The listing builds one solid part. Answer for the finished solid, in the listing's coordinates (mm). Face numbers are marked on the shaded views. A direction names the side the tool comes from. Round coordinates to 2 decimals unless told otherwise and drop trailing zeros. Loops run counter-clockwise (first coordinate to the right, second up) from the corner with the lowest first, then second, coordinate; pieces in that order, holes last. Notation, with made-up numbers: (51, 73) -> (86, 73) arc R16 cw to (86, 98) -> close; hole circle Ø5 at (-34.5, 19). An arc over 180 degrees is marked (long way). Use a Markdown table: item, result. Add a question column.
Q1. Which of the six approach directions +Z, -Z, +X, -X, +Y, -Y give full straight-line access (tool end or side, diameter ignored) to the marked faces 4, 5, 6 and 7?
Q2. Section C-C on x = 8 is taken. Give the vertices of the cut face in (y, z).
Q3. Section A-A on x = 0 is taken. Give the vertices of the cut face in (y, z).
Q4. For a pull along X with two mould halves and no side action, classify the marked faces 1, 2 and 3 as released by +X, released by -X, zero draft, split by the parting line, or undercut.
Q5. Section D-D on x = 3.75 is taken. Give the vertices of the cut face in (y, z).
Q6. Consider line 1 (X direction, y = 2.55, z = 14); line 2 (X direction, y = 0.85, z = 9.75); line 3 (Z direction, x = 0, y = 2.45). Determine where each line is inside the solid, lowest interval first.
Q7. Section B-B on y = 2.3 is taken. Give the vertices of the cut face in (x, z), then the cut area to 3 significant figures.
Q8. Given pin 1 Ø1.2 at (x, y) = (11.5, 1.5) entering from +Z; pin 2 Ø0.9 at (y, z) = (1, 13.5) entering from +X; pin 3 Ø0.6 at (x, y) = (0.5, 1) entering from +Z, each flat-ended and moving along its own axis, determine where each tip first touches the part or whether it passes through.
from build123d import *

# Parameters (mm, degrees)
BOSS_EXTRUDE1_DEPTH = 3
SKETCH3_R           = 1.5
CUT_EXTRUDE1_DEPTH  = 3
FILLET1_R           = 2
SKETCH4_R           = 1
CUT_EXTRUDE2_DEPTH  = 10


with BuildPart() as part:
    # Sketch2 → Boss-Extrude1 (new body)
    with BuildSketch(Plane(origin=(0, 0, 0), x_dir=(1, 0, 0), z_dir=(0, 1, 0))):
        with BuildLine():
            Line((4.668611776, -14.59443044), (4.668611776, -22.09443044))
            ThreePointArc((4.668611776, -22.09443044), (7.568611776, -24.99443044), (10.468611776, -22.09443044))
            Line((10.468611776, -22.09443044), (10.468611776, -14.59443044))
            Line((10.468611776, -14.59443044), (10.468611776, -10.59443044))
            Line((10.468611776, -10.59443044), (11.968611776, -10.59443044))
            Line((11.968611776, -10.59443044), (11.968611776, -5.761851858))
            ThreePointArc((11.968611776, -5.761851858), (7.254363967, -4.368466387), (5, 0))
            ThreePointArc((5, 0), (0, 5), (-5, 0))
            ThreePointArc((-5, 0), (-7.028472422, -4.339612176), (-11.531388224, -5.973834769))
            Line((-11.531388224, -5.973834769), (-11.531388224, -10.806413351))
            Line((-11.531388224, -10.806413351), (-10.031388224, -10.806413351))
            Line((-10.031388224, -10.806413351), (-10.031388224, -14.806413351))
            Line((-10.031388224, -14.806413351), (-4.231388224, -14.806413351))
            Line((-4.231388224, -14.806413351), (-4.231388224, -10.806413351))
            Line((-4.231388224, -10.806413351), (-0.781388224, -10.806413351))
            Line((-0.781388224, -10.806413351), (-0.781388224, -6.306413351))
            Line((-0.781388224, -6.306413351), (1.218611776, -6.306413351))
            Line((1.218611776, -6.306413351), (1.218611776, -10.806413351))
            Line((1.218611776, -10.806413351), (4.668611776, -10.806413351))
            Line((4.668611776, -10.806413351), (4.668611776, -14.59443044))
        make_face()
    extrude(amount=BOSS_EXTRUDE1_DEPTH)

    # Sketch3 → Cut-Extrude1 (cut)
    with BuildSketch(Plane(origin=(0, 3, 0), x_dir=(1, 0, 0), z_dir=(0, 1, 0))):
        Circle(SKETCH3_R)
    extrude(amount=-CUT_EXTRUDE1_DEPTH, mode=Mode.SUBTRACT)

    # Fillet1
    fillet1_edges = [part.edges().sort_by_distance(p)[0] for p in [
        (-11.531388224, 1.5, 5.973834769),
        (11.968611776, 1.5, 5.761851858),
    ]]
    fillet(fillet1_edges, radius=FILLET1_R)

    # Sketch4 → Cut-Extrude2 (cut)
    with BuildSketch(Plane(origin=(0, 3, 0), x_dir=(1, 0, 0), z_dir=(0, 1, 0))):
        with Locations((7.568611776, -22.09443044)):
            Circle(SKETCH4_R)
    extrude(amount=-CUT_EXTRUDE2_DEPTH, mode=Mode.SUBTRACT)


solid = part.part
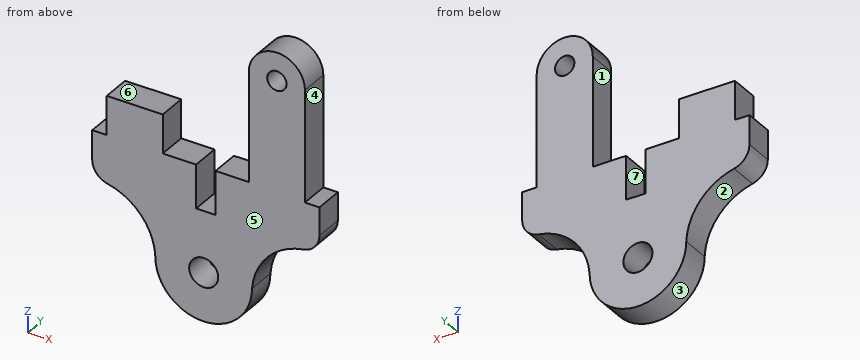
Checked values:
| question | item | result |
|---|---|---|
| 1 | face 4 | +Z, +X, +Y, -Y |
| 1 | face 5 | +Z, -Z, +X, -X, -Y |
| 1 | face 6 | +Z, -X, +Y, -Y |
| 1 | face 7 | +Z, +Y, -Y |
| 2 | outline | (0, 4.9) -> (3, 4.9) -> (3, 21.19) -> (0, 21.19) -> close; (0, 23) -> (3, 23) -> (3, 24.96) -> (0, 24.96) -> close |
| 3 | outline | (0, -5) -> (3, -5) -> (3, -1.5) -> (0, -1.5) -> close; (0, 1.5) -> (3, 1.5) -> (3, 6.31) -> (0, 6.31) -> close |
| 4 | face 1 | undercut |
| 4 | face 2 | released by -X |
| 4 | face 3 | split by the parting line |
| 5 | outline | (0, -3.31) -> (3, -3.31) -> (3, 10.81) -> (0, 10.81) -> close |
| 6 | line 1 | x = -10.03 to -4.23, 4.67 to 10.47 |
| 6 | line 2 | x = -11.53 to -0.78, 1.22 to 11.97 |
| 6 | line 3 | z = -5 to -1.5, 1.5 to 6.31 |
| 7 | outline | (-11.53, 7.8) arc R2 ccw to (-9.95, 5.84) arc R6.26 cw to (-5, 0) arc R5 ccw to (5, 0) arc R6.26 cw to (10.28, 5.73) arc R2 ccw to (11.97, 7.71) -> (11.97, 10.59) -> (10.47, 10.59) -> (10.47, 22.09) arc R2.9 ccw to (4.67, 22.09) -> (4.67, 10.81) -> (1.22, 10.81) -> (1.22, 6.31) -> (-0.78, 6.31) -> (-0.78, 10.81) -> (-4.23, 10.81) -> (-4.23, 14.81) -> (-10.03, 14.81) -> (-10.03, 10.81) -> (-11.53, 10.81) -> close; hole circle Ø3 at (0, 0); hole circle Ø2 at (7.57, 22.09) |
| 7 | area | 311 mm2 |
| 8 | pin 1 | stops at z = 10.59 |
| 8 | pin 2 | stops at x = 10.47 |
| 8 | pin 3 | stops at z = 6.31 |
